Source: CAD feature listing. Evaluate the final solid. Frame: model axes, mm. A direction names the side the tool comes from. Coordinates: 2 decimals unless noted, no trailing zeros. Order: outer loops, then holes, each group sorted by start corner. A loop starts at its lowest first (then second) coordinate and runs counter-clockwise, first axis right, second up. Notation, with made-up numbers: (19, -14) - (59, -14) arc R11 cw to (59, -9) - close; hole circle Ø7 at (76.5, 84.5). An arc over 180 degrees is marked (long way). One line per question, with ' | ' between items.
from build123d import *

# Parameters (mm, degrees)
SKETCH1_R           = 1.651
SKETCH1_W           = 25.4
SKETCH1_H           = 50.8
BOSS_EXTRUDE1_DEPTH = 3.175


with BuildPart() as part:
    # Sketch1 → Boss-Extrude1 (new body)
    with BuildSketch(Plane(origin=(0, 0, 0), x_dir=(1, 0, 0), z_dir=(0, 1, 0))):
        with BuildLine():
            Line((-73.916912814, 12.7), (-73.916912814, -12.7))
            ThreePointArc((-73.916912814, -12.7), (-67.357563081, -32.984218889), (-55.35602635, -50.603461806))
            Line((-55.35602635, -50.603461806), (55.35602635, -50.603461806))
            ThreePointArc((55.35602635, -50.603461806), (75, 0), (55.35602635, 50.603461806))
            Line((55.35602635, 50.603461806), (-55.35602635, 50.603461806))
            ThreePointArc((-55.35602635, 50.603461806), (-67.357563081, 32.984218889), (-73.916912814, 12.7))
        make_face()
        with Locations(Location((13.713087186, 34.29, 0), (0, 0, 270))):
            Circle(SKETCH1_R, mode=Mode.SUBTRACT)
        with Locations(Location((-58.676912814, -34.29, 0), (0, 0, 270))):
            Circle(SKETCH1_R, mode=Mode.SUBTRACT)
        with Locations(Location((-58.676912814, 34.29, 0), (0, 0, 270))):
            Circle(SKETCH1_R, mode=Mode.SUBTRACT)
        with Locations(Location((-39.626912814, 47.428461806, 0), (0, 0, 270))):
            Circle(SKETCH1_R, mode=Mode.SUBTRACT)
        with Locations(Location((51.749406285, 47.428461806, 0), (0, 0, 270))):
            Circle(SKETCH1_R, mode=Mode.SUBTRACT)
        with Locations(Location((-39.626912814, -47.428461806, 0), (0, 0, 270))):
            Circle(SKETCH1_R, mode=Mode.SUBTRACT)
        with Locations(Location((51.749406285, -47.428461806, 0), (0, 0, 270))):
            Circle(SKETCH1_R, mode=Mode.SUBTRACT)
        with Locations(Location((56.893087186, 34.29, 0), (0, 0, 270))):
            Circle(SKETCH1_R, mode=Mode.SUBTRACT)
        with Locations(Location((-48.516912814, 34.29, 0), (0, 0, 270))):
            Circle(SKETCH1_R, mode=Mode.SUBTRACT)
        with Locations(Location((-5.336912814, 34.29, 0), (0, 0, 270))):
            Circle(SKETCH1_R, mode=Mode.SUBTRACT)
        with Locations(Location((-5.336912814, -34.29, 0), (0, 0, 270))):
            Circle(SKETCH1_R, mode=Mode.SUBTRACT)
        with Locations(Location((-48.516912814, -34.29, 0), (0, 0, 270))):
            Circle(SKETCH1_R, mode=Mode.SUBTRACT)
        with Locations(Location((13.713087186, -34.29, 0), (0, 0, 270))):
            Circle(SKETCH1_R, mode=Mode.SUBTRACT)
        with Locations(Location((56.893087186, -34.29, 0), (0, 0, 270))):
            Circle(SKETCH1_R, mode=Mode.SUBTRACT)
        Rectangle(SKETCH1_W, SKETCH1_H, mode=Mode.SUBTRACT)
    extrude(amount=BOSS_EXTRUDE1_DEPTH)


solid = part.part
(1) Material intervals for L1, parallel to Z at x = 51, y = 2.8; L2, parallel to X at y = 2.2, z = 34.29; L3, parallel to Z at x = 1.5, y = 2.85, sorted ascending. Write a range as from..to.
Taken from the geometry:
L1: z = -50.6..-48.9, -45.96..45.96, 48.9..50.6 | L2: x = -66.7..-60.33, -57.03..-50.17, -46.87..-6.99, -3.69..12.06, 15.36..55.24, 58.54..66.7 | L3: z = -50.6..-25.4, 25.4..50.6
(2) Cut plane B-B (y = 0.9). State how many separate pieces and enclosed holes the cut face has, and give its area (3 significant figures).
Taken from the geometry:
separate pieces: 1 | enclosed holes: 15 | area: 12,500 mm²
(3) Cut plane C-C (z = -34.29). Return the cut outline in (x, y) (3 decimals), and give its area (3 significant figures).
Taken from the geometry:
outline: (-66.702, 0) - (-60.328, 0) - (-60.328, 3.175) - (-66.702, 3.175) - close; (-57.026, 0) - (-50.168, 0) - (-50.168, 3.175) - (-57.026, 3.175) - close; (-46.866, 0) - (-6.988, 0) - (-6.988, 3.175) - (-46.866, 3.175) - close; (-3.686, 0) - (12.062, 0) - (12.062, 3.175) - (-3.686, 3.175) - close; (15.364, 0) - (55.242, 0) - (55.242, 3.175) - (15.364, 3.175) - close; (58.544, 0) - (66.702, 0) - (66.702, 3.175) - (58.544, 3.175) - close | area: 371 mm²
(4) Set-up query: faces 4 (the cylindrical face through (-67.2, 1.6, -33.3)), 5 (the flat face through (0, 2, 25.4)). Return all of +Z, -Z, +X, -X, +Y, -Y with unobstructed straight access to the full face (end or side cutting, diameter ignored); none if empty.
Taken from the geometry:
face 4: -Z, -X, +Y, -Y | face 5: +Y, -Y
(5) Pin query (flat end, axial travel): P1, Ø2.5, axis at x = -5.34, z = -34.29, coming from the +Y side; P2, Ø5.5, axis at x = 51.75, z = -47.43, coming from the +Y side (3 decimals); P3, Ø1, axis at y = 1, z = -4, coming from the +X side. Return the tip coordinate at first contact, or that it passes through.
Taken from the geometry:
P1: passes through | P2: stops at y = 3.175 | P3: stops at x = 74.92
(6) Cut plane A-A (x = 3.5). Return the cut outline in (y, z) (3 decimals), and give its area (3 significant figures).
Taken from the geometry:
outline: (0, -50.603) - (3.175, -50.603) - (3.175, -25.4) - (0, -25.4) - close; (0, 25.4) - (3.175, 25.4) - (3.175, 50.603) - (0, 50.603) - close | area: 160 mm²
(7) Pull-direction query (X, two-part tool) for faces 1 (the flat face through (-73.917, 2, 0)), 2 (the flat face through (16, 3.175, -1)), 3 (the flat face through (0, 2, -25.4)); classes: pulls with the +X half, pulls with the -X half, needs draft (parallel to the pull), parting line crosses it, or undercut.
Taken from the geometry:
face 1: pulls with the -X half | face 2: needs draft | face 3: undercut
(8) Cut plane D-D (z = 9.5). Return the cut outline in (x, y) (3 decimals).
Taken from the geometry:
outline: (-73.917, 0) - (-12.7, 0) - (-12.7, 3.175) - (-73.917, 3.175) - close; (12.7, 0) - (74.396, 0) - (74.396, 3.175) - (12.7, 3.175) - close
